Input: part model. Units: mm. Frame: model coordinates. Give positions to 0.01 mm unless a question says otherwise; leave off trailing zeros. Loops run counter-clockwise (first coordinate to the right, second up) from the corner with the lowest first, then second, coordinate; pieces in that order, holes last. Notation, with made-up numbers: (-11.75, -12.5) - (-7.75, -12.5) arc R12 cw to (-7.75, 0.5) - close; hole circle Ø11 at (29.25, -28.75). An arc over 180 degrees is marked (long way). Answer as a JSON object with one key per item and string values.
from build123d import *

# Parameters (mm, degrees)
F1_DEPTH = 1.5
F2_R     = 5
F3_R     = 2
F3_R_2   = 1.965178389
F3_R_3   = 2.0701414228
F3_R_4   = 1.9676743652
F4_DEPTH = 25


# Not quite as in the source:
# - a feature names something its author has since deleted; it is built from what else it names


with BuildPart() as f1:
    # F0 (on Front) → F1 (new body, symmetric)
    with BuildSketch(Plane.XZ):
        Polygon((-44.9992595649, -10.2426138069), (45.0007404351, -9.7573861383), (44.9992595649, 10.2426138069), (-35.7811990629, 9.8070925446), align=None)
    extrude(amount=F1_DEPTH, both=True)

    # F2
    f2_edges = [f1.edges().sort_by_distance(p)[0] for p in [
        (45.00074, 0, -9.757386),
        (-35.781199, 0, 9.807093),
        (-44.99926, 0, -10.242614),
        (44.99926, 0, 10.242614),
    ]]
    fillet(f2_edges, radius=F2_R)

    # F3 (on face) → F4 (cut)
    with BuildSketch(Plane.XZ.offset(1.5)):
        with Locations((37.9996325629, 5.2048032201)):
            Circle(F3_R)
        with Locations((27.9996325629, 5.1508890347)):
            Circle(F3_R)
        with Locations((17.9996325629, 5.0969748493)):
            Circle(F3_R_2)
        with Locations((7.9996325629, 5.0430606639)):
            Circle(F3_R_2)
        with Locations((-2.0003674371, 4.9891464785)):
            Circle(F3_R_3)
        with Locations((-12.0003674371, 4.9352322931)):
            Circle(F3_R_3)
        with Locations((-22.0003674371, 4.8813181077)):
            Circle(F3_R_4)
        with Locations((38.0535444404, -4.7947687116)):
            Circle(F3_R)
        with Locations((28.0535444404, -4.848682897)):
            Circle(F3_R)
        with Locations((18.0535444404, -4.9025970824)):
            Circle(F3_R)
        with Locations((8.0535444404, -4.9565112678)):
            Circle(F3_R)
        with Locations((0, -4.9999312966)):
            Circle(F3_R)
        with Locations((-11.9464555596, -5.0643396386)):
            Circle(F3_R)
        with Locations((-21.9464555596, -5.118253824)):
            Circle(F3_R)
        with Locations((-32.0003674371, -5.1724586709)):
            Circle(F3_R)
    extrude(amount=-F4_DEPTH, mode=Mode.SUBTRACT)


solid = f1.part
Item 1: Cut plane B-B (y = -0.4). Give the number of separate pieces and of enclosed holes in the cut face, then the cut area to 3 significant figures.
Geometry check:
{"separate pieces": "1", "enclosed holes": "15", "area": "1,490 mm2"}
Item 2: Cut plane A-A (x = -21.5). Return loops of the section in (y, z).
Geometry check:
{"outline": "(-1.5, -10.12) - (1.5, -10.12) - (1.5, -7.07) - (-1.5, -7.07) - close; (-1.5, -3.17) - (1.5, -3.17) - (1.5, 2.98) - (-1.5, 2.98) - close; (-1.5, 6.78) - (1.5, 6.78) - (1.5, 9.88) - (-1.5, 9.88) - close"}
Item 3: Mould query, pull axis Z, two halves, no side actions, for faces 1 (the face through (-35.311, 0.021, 9.005)), 2 (the face through (43.507, -0.021, -8.349)), 3 (the face through (-0.887, -0.021, 6.735)). Classes: released by +Z, released by -Z, zero draft, split by the parting line, or undercut.
Geometry check:
{"face 1": "released by +Z", "face 2": "released by -Z", "face 3": "undercut"}
Item 4: Material intervals for line 1 (Z direction, x = 18.5, y = 0.1); line 2 (Z direction, x = 7.5, y = 0.3); line 3 (X direction, y = 1.2, z = -8), sorted ascending. Write a range as [from, to].
Geometry check:
{"line 1": "z = [-9.9, -6.85], [-2.95, 3.2], [7, 10.1]", "line 2": "z = [-9.96, -6.88], [-3.03, 3.14], [6.94, 10.04]", "line 3": "x = [-41.32, 43.83]"}
Item 5: Cut plane D-D (x = 31). Return loops of the section in (y, z), then the cut area to 3 significant figures.
Geometry check:
{"outline": "(-1.5, -9.83) - (1.5, -9.83) - (1.5, 10.17) - (-1.5, 10.17) - close", "area": "60.0 mm2"}
Item 6: Cut plane C-C (z = 1.5). Return loops of the section in (x, y), then the cut area to 3 significant figures.
Geometry check:
{"outline": "(-39.6, -1.5) - (45, -1.5) - (45, 1.5) - (-39.6, 1.5) - close", "area": "254 mm2"}
Item 7: Contact query for a flat-ended pin moving along its axis: P1, Ø1.5, axis at x = -1.5, y = -1, coming from the +Z side. Output: stop coordinate, or through.
Geometry check:
{"P1": "stops at z = 10"}
